The listing builds one solid part. Answer for the finished solid, in the listing's coordinates (mm). Face numbers are marked on the shaded views. A direction names the side the tool comes from. Coordinates: 2 decimals unless noted, no trailing zeros. Write each loop counter-clockwise with the first axis right and the second up, starting at its lowest first coordinate (ties: lowest second). Pieces come first, ordered by that corner, then holes.
(1) Which of the six approach directions +Z, -Z, +X, -X, +Y, -Y give full straight-line access (tool end or side, diameter ignored) to the marked faces 4, 5, 6 and 7?
(2) Given P1, Ø0.9, axis at x = 16, z = 108, coming from the -Y side; P2, Ø14.5, axis at x = -8.62, y = -7.1, coming from the +Z side; P3, Ø2, axis at x = -10.5, y = 6, coming from the +Z side, each flat-ended and moving along its own axis, determine where each tip first touches the part or whether it passes through.
(3) The part is cut by section C-C on z = 126. Determine the outline of the cut face in (x, y).
(4) Straight lines are drawn through the part: line 1 (Z direction, x = 7.5, y = -4); line 2 (X direction, y = -20.5, z = 135.5); line 3 (X direction, y = -4, z = 112). For each, find the intervals that lie inside material, in ascending order.
(5) The part is cut by section D-D on y = -18.5. Determine the outline of the cut face in (x, z).
(6) For a pull along Y with two mould halves and no side action, classify the marked faces 1, 2 and 3 as +Y half, -Y half, draft (parallel to the pull), parting line (faces both ways), or undercut.
(7) The part is cut by section B-B on x = -27.5. Determine the outline of the cut face in (y, z) (3 decimals), plus the area to 3 significant figures.
(8) The part is cut by section A-A on x = 13.5. Determine the outline of the cut face in (y, z).
from build123d import *

# Parameters (mm, degrees)
SALIENTE_EXTRUIR1_START = 2.5
SALIENTE_EXTRUIR1_DEPTH = 5
CROQUIS2_R              = 13.5
CORTAR_EXTRUIR1_DEPTH   = 3.5
CROQUIS4_R              = 4.025
SALIENTE_EXTRUIR3_DEPTH = 9
CROQUIS5_W              = 5
CROQUIS5_H              = 36
SALIENTE_EXTRUIR4_DEPTH = 38.35
CORTAR_EXTRUIR2_DEPTH   = 2
CROQUIS8_R              = 4.55
CORTAR_EXTRUIR3_DEPTH   = 67.15821583
SALIENTE_EXTRUIR5_DEPTH = 5
CORTAR_EXTRUIR4_DEPTH   = 5
SALIENTE_EXTRUIR6_START = 3.65
CROQUIS12_R             = 1
SALIENTE_EXTRUIR6_DEPTH = 3.65
SALIENTE_EXTRUIR7_START = -8.65
SALIENTE_EXTRUIR7_DEPTH = 8.65
CROQUIS14_R             = 1
CORTAR_EXTRUIR5_DEPTH   = 3.65
CROQUIS15_W             = 7.15
CROQUIS15_H             = 2.35
CORTAR_EXTRUIR6_DEPTH   = 2
CROQUIS16_W             = 7.15
CROQUIS16_H             = 2.35
SALIENTE_EXTRUIR8_DEPTH = 2
SALIENTE_EXTRUIR9_START = 2.15
CROQUIS17_R             = 1
SALIENTE_EXTRUIR9_DEPTH = 2.15
CROQUIS18_W             = 55
CROQUIS18_H             = 3
CORTAR_EXTRUIR7_DEPTH   = 3


with BuildPart() as part:
    # Croquis1 → Saliente-Extruir1 (new body)
    with BuildSketch(Plane.ZY.offset(28.973126084).offset(SALIENTE_EXTRUIR1_START)):
        with BuildLine():
            Line((108.890000566, 10.898170258), (108.890000566, -25.101829742))
            Line((108.890000566, -25.101829742), (143.890000566, -22.601829742))
            ThreePointArc((143.890000566, -22.601829742), (159.390000566, -7.101829742), (143.890000566, 8.398170258))
            Line((143.890000566, 8.398170258), (108.890000566, 10.898170258))
        make_face()
    extrude(amount=-SALIENTE_EXTRUIR1_DEPTH)

    # Croquis2 → Cortar-Extruir1 (cut)
    with BuildSketch(Plane(origin=(-26.473126084, 0, 0), x_dir=(0, 0, -1), z_dir=(1, 0, 0))):
        with Locations((-143.890000566, -7.101829742)):
            Circle(CROQUIS2_R)
    extrude(amount=-CORTAR_EXTRUIR1_DEPTH, mode=Mode.SUBTRACT)

    # Croquis4 → Saliente-Extruir3 (add)
    with BuildSketch(Plane(origin=(-29.973126084, 0, 0), x_dir=(0, 0, -1), z_dir=(1, 0, 0))):
        with Locations(Location((-143.890000566, -7.101829742, 0), (0, 0, 180))):
            Circle(CROQUIS4_R)
    extrude(amount=SALIENTE_EXTRUIR3_DEPTH)

    # Croquis5 → Saliente-Extruir4 (add)
    with BuildSketch(Plane.ZY.offset(31.473126084)):
        with Locations((106.390000566, -7.101829742)):
            Rectangle(CROQUIS5_W, CROQUIS5_H)
    extrude(amount=-SALIENTE_EXTRUIR4_DEPTH)

    # Croquis6 → Cortar-Extruir2 (cut)
    with BuildSketch(Plane.XY.offset(108.890000566)):
        with BuildLine():
            Line((-21.743906953, -10.757089493), (-16.168906615, -6.706372141))
            Line((-16.168906615, -6.706372141), (-21.289951258, -2.095098824))
            ThreePointArc((-21.289951258, -2.095098824), (-22.060016072, 1.624188646), (-18.349064321, 2.433469933))
            Line((-18.349064321, 2.433469933), (-12.053540021, -0.36926331))
            Line((-12.053540021, -0.36926331), (-10.620582506, 6.371328103))
            ThreePointArc((-10.620582506, 6.371328103), (-7.784617481, 8.89786753), (-5.228283452, 6.088729685))
            Line((-5.228283452, 6.088729685), (-4.50775949, -0.764720911))
            Line((-4.50775949, -0.764720911), (2.046242668, 1.364597186))
            ThreePointArc((2.046242668, 1.364597186), (5.652272507, 0.171849142), (4.497654785, -3.44656999))
            Line((4.497654785, -3.44656999), (-1.077345553, -7.497287342))
            Line((-1.077345553, -7.497287342), (4.04369909, -12.108560659))
            ThreePointArc((4.04369909, -12.108560659), (4.813763904, -15.827848129), (1.102812153, -16.637129416))
            Line((1.102812153, -16.637129416), (-5.192712147, -13.834396173))
            Line((-5.192712147, -13.834396173), (-6.625669661, -20.574987586))
            ThreePointArc((-6.625669661, -20.574987586), (-9.461634687, -23.101527013), (-12.017968716, -20.292389168))
            Line((-12.017968716, -20.292389168), (-12.738492677, -13.438938572))
            Line((-12.738492677, -13.438938572), (-19.292494835, -15.568256669))
            ThreePointArc((-19.292494835, -15.568256669), (-22.898524675, -14.375508625), (-21.743906953, -10.757089493))
        make_face()
    extrude(amount=-CORTAR_EXTRUIR2_DEPTH, mode=Mode.SUBTRACT)

    # Croquis8 → Cortar-Extruir3 (cut, through all)
    with BuildSketch(Plane.XY.offset(106.890000566)):
        with Locations((-8.623126084, -7.101829742)):
            Circle(CROQUIS8_R)
    extrude(amount=-CORTAR_EXTRUIR3_DEPTH, mode=Mode.SUBTRACT)

    # Croquis9 → Saliente-Extruir5 (add)
    with BuildSketch(Plane(origin=(6.876873916, 0, 0), x_dir=(0, 0, -1), z_dir=(1, 0, 0))):
        with BuildLine():
            Line((-143.890000566, -22.601829742), (-108.890000566, -25.101829742))
            Line((-108.890000566, -25.101829742), (-103.890000566, -25.101829742))
            Line((-103.890000566, -25.101829742), (-103.890000566, 10.898170258))
            Line((-103.890000566, 10.898170258), (-108.890000566, 10.898170258))
            Line((-108.890000566, 10.898170258), (-143.890000566, 8.398170258))
            ThreePointArc((-143.890000566, 8.398170258), (-159.390000566, -7.101829742), (-143.890000566, -22.601829742))
        make_face()
    extrude(amount=SALIENTE_EXTRUIR5_DEPTH)

    # Croquis11 → Cortar-Extruir4 (cut)
    with BuildSketch(Plane(origin=(11.876873916, 0, 0), x_dir=(0, 0, -1), z_dir=(1, 0, 0))):
        with BuildLine():
            Line((-153.240000566, 1.898170258), (-153.240000566, -16.101829742))
            ThreePointArc((-153.240000566, -16.101829742), (-152.844594721, -17.056423896), (-151.890000566, -17.451829742))
            Line((-151.890000566, -17.451829742), (-113.890000566, -17.451829742))
            ThreePointArc((-113.890000566, -17.451829742), (-112.935406411, -17.056423896), (-112.540000566, -16.101829742))
            Line((-112.540000566, -16.101829742), (-112.540000566, 1.898170258))
            ThreePointArc((-112.540000566, 1.898170258), (-112.935406411, 2.852764413), (-113.890000566, 3.248170258))
            Line((-113.890000566, 3.248170258), (-151.890000566, 3.248170258))
            ThreePointArc((-151.890000566, 3.248170258), (-152.844594721, 2.852764413), (-153.240000566, 1.898170258))
        make_face()
    extrude(amount=-CORTAR_EXTRUIR4_DEPTH, mode=Mode.SUBTRACT)

    # Croquis12 → Saliente-Extruir6 (add)
    with BuildSketch(Plane(origin=(11.876873916, 0, 0), x_dir=(0, 0, -1), z_dir=(1, 0, 0)).offset(SALIENTE_EXTRUIR6_START)):
        with BuildLine():
            Line((-105.390000566, -1.251829742), (-105.390000566, -3.951829742))
            Line((-105.390000566, -3.951829742), (-105.390000566, -10.251829742))
            Line((-105.390000566, -10.251829742), (-105.390000566, -12.951829742))
            Line((-105.390000566, -12.951829742), (-105.390000566, -13.601829742))
            ThreePointArc((-105.390000566, -13.601829742), (-106.268680223, -15.723150085), (-108.390000566, -16.601829742))
            Line((-108.390000566, -16.601829742), (-112.636006946, -16.601829742))
            ThreePointArc((-112.636006946, -16.601829742), (-112.564219402, -16.356396641), (-112.540000566, -16.101829742))
            Line((-112.540000566, -16.101829742), (-112.540000566, 1.898170258))
            ThreePointArc((-112.540000566, 1.898170258), (-112.564219402, 2.152737158), (-112.636006946, 2.398170258))
            Line((-112.636006946, 2.398170258), (-108.390000566, 2.398170258))
            ThreePointArc((-108.390000566, 2.398170258), (-106.268680223, 1.519490602), (-105.390000566, -0.601829742))
            Line((-105.390000566, -0.601829742), (-105.390000566, -1.251829742))
        make_face()
        with Locations((-107.494163107, -2.601829742)):
            Circle(CROQUIS12_R, mode=Mode.SUBTRACT)
        with Locations((-107.494163107, -11.601829742)):
            Circle(CROQUIS12_R, mode=Mode.SUBTRACT)
    extrude(amount=-SALIENTE_EXTRUIR6_DEPTH)

    # Croquis13 → Saliente-Extruir7 (add)
    with BuildSketch(Plane.ZY.offset(-6.876873916).offset(SALIENTE_EXTRUIR7_START)):
        with BuildLine():
            Line((153.240000566, -16.101829742), (153.240000566, 1.898170258))
            ThreePointArc((153.240000566, 1.898170258), (153.21578173, 2.152737158), (153.143994186, 2.398170258))
            Line((153.143994186, 2.398170258), (157.390000566, 2.398170258))
            ThreePointArc((157.390000566, 2.398170258), (159.51132091, 1.519490602), (160.390000566, -0.601829742))
            Line((160.390000566, -0.601829742), (160.390000566, -1.251829742))
            Line((160.390000566, -1.251829742), (160.390000566, -3.951829742))
            Line((160.390000566, -3.951829742), (160.390000566, -10.251829742))
            Line((160.390000566, -10.251829742), (160.390000566, -12.951829742))
            Line((160.390000566, -12.951829742), (160.390000566, -13.601829742))
            ThreePointArc((160.390000566, -13.601829742), (159.51132091, -15.723150085), (157.390000566, -16.601829742))
            Line((157.390000566, -16.601829742), (153.143994186, -16.601829742))
            ThreePointArc((153.143994186, -16.601829742), (153.21578173, -16.356396641), (153.240000566, -16.101829742))
        make_face()
    extrude(amount=SALIENTE_EXTRUIR7_DEPTH)

    # Croquis14 → Cortar-Extruir5 (cut)
    with BuildSketch(Plane(origin=(15.526873916, 0, 0), x_dir=(0, 0, -1), z_dir=(1, 0, 0))):
        with Locations((-158.285838025, -2.601829742)):
            Circle(CROQUIS14_R)
        with Locations((-158.285838025, -11.601829742)):
            Circle(CROQUIS14_R)
    extrude(amount=-CORTAR_EXTRUIR5_DEPTH, mode=Mode.SUBTRACT)

    # Croquis15 → Cortar-Extruir6 (cut)
    with BuildSketch(Plane(origin=(15.526873916, 0, 0), x_dir=(0, 0, -1), z_dir=(1, 0, 0))):
        with Locations((-108.965000566, -7.101829742)):
            Rectangle(CROQUIS15_W, CROQUIS15_H)
        with Locations((-156.815000566, -7.101829742)):
            Rectangle(CROQUIS15_W, CROQUIS15_H)
    extrude(amount=-CORTAR_EXTRUIR6_DEPTH, mode=Mode.SUBTRACT)

    # Croquis16 → Saliente-Extruir8 (add)
    with BuildSketch(Plane(origin=(13.526873916, 0, 0), x_dir=(0, 0, -1), z_dir=(1, 0, 0))):
        with Locations((-156.815000566, -7.101829742)):
            Rectangle(CROQUIS16_W, CROQUIS16_H)
        with Locations((-108.965000566, -7.101829742)):
            Rectangle(CROQUIS16_W, CROQUIS16_H)
    extrude(amount=SALIENTE_EXTRUIR8_DEPTH)

    # Croquis17 → Saliente-Extruir9 (add)
    # profile 1 of 2: a face of its own
    with BuildSketch(Plane(origin=(15.526873916, 0, 0), x_dir=(0, 0, -1), z_dir=(1, 0, 0)).offset(SALIENTE_EXTRUIR9_START)):
        with BuildLine():
            Line((-105.390000566, -13.601829742), (-105.390000566, -0.601829742))
            ThreePointArc((-105.390000566, -0.601829742), (-106.268680223, 1.519490602), (-108.390000566, 2.398170258))
            Line((-108.390000566, 2.398170258), (-112.636006946, 2.398170258))
            ThreePointArc((-112.636006946, 2.398170258), (-112.564219402, 2.152737158), (-112.540000566, 1.898170258))
            Line((-112.540000566, 1.898170258), (-112.540000566, -16.101829742))
            ThreePointArc((-112.540000566, -16.101829742), (-112.564219402, -16.356396641), (-112.636006946, -16.601829742))
            Line((-112.636006946, -16.601829742), (-108.390000566, -16.601829742))
            ThreePointArc((-108.390000566, -16.601829742), (-106.268680223, -15.723150085), (-105.390000566, -13.601829742))
        make_face()
        with Locations((-107.494163107, -11.601829742)):
            Circle(CROQUIS17_R, mode=Mode.SUBTRACT)
        with Locations((-107.494163107, -2.601829742)):
            Circle(CROQUIS17_R, mode=Mode.SUBTRACT)
    # profile 2 of 2: a face of its own
    with BuildSketch(Plane(origin=(15.526873916, 0, 0), x_dir=(0, 0, -1), z_dir=(1, 0, 0)).offset(SALIENTE_EXTRUIR9_START)):
        with BuildLine():
            Line((-160.390000566, -0.601829742), (-160.390000566, -13.601829742))
            ThreePointArc((-160.390000566, -13.601829742), (-159.51132091, -15.723150085), (-157.390000566, -16.601829742))
            Line((-157.390000566, -16.601829742), (-153.143994186, -16.601829742))
            ThreePointArc((-153.143994186, -16.601829742), (-153.21578173, -16.356396641), (-153.240000566, -16.101829742))
            Line((-153.240000566, -16.101829742), (-153.240000566, 1.898170258))
            ThreePointArc((-153.240000566, 1.898170258), (-153.21578173, 2.152737158), (-153.143994186, 2.398170258))
            Line((-153.143994186, 2.398170258), (-157.390000566, 2.398170258))
            ThreePointArc((-157.390000566, 2.398170258), (-159.51132091, 1.519490602), (-160.390000566, -0.601829742))
        make_face()
        with Locations((-158.285838025, -11.601829742)):
            Circle(CROQUIS17_R, mode=Mode.SUBTRACT)
        with Locations((-158.285838025, -2.601829742)):
            Circle(CROQUIS17_R, mode=Mode.SUBTRACT)
    extrude(amount=-SALIENTE_EXTRUIR9_DEPTH)

    # Croquis18 → Cortar-Extruir7 (cut)
    with BuildSketch(Plane(origin=(17.676873916, 0, 0), x_dir=(0, 0, -1), z_dir=(1, 0, 0))):
        with Locations((-132.890000566, -7.101829742)):
            Rectangle(CROQUIS18_W, CROQUIS18_H)
    extrude(amount=-CORTAR_EXTRUIR7_DEPTH, mode=Mode.SUBTRACT)


solid = part.part
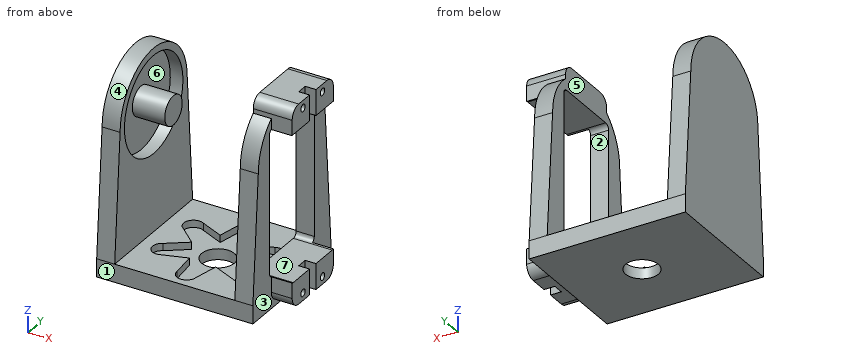
Model answer:
1. face 4: +Z, -X
1. face 5: +Z, +Y, -Y
1. face 6: none
1. face 7: +X
2. P1: stops at y = -16.6
2. P2: stops at z = 106.89
2. P3: stops at z = 108.89
3. outline: (-31.47, -23.88) - (-26.47, -23.88) - (-26.47, 9.68) - (-31.47, 9.68) - close; (6.88, -23.88) - (11.88, -23.88) - (11.88, -17.45) - (6.88, -17.45) - close; (6.88, 3.25) - (11.88, 3.25) - (11.88, 9.68) - (6.88, 9.68) - close
4. line 1: z = 103.89 to 112.54, 153.24 to 160.39
4. line 2: x = -31.47 to -26.47, 6.88 to 11.88
4. line 3: x = -31.47 to -26.47, 6.88 to 17.68
5. outline: (-31.47, 103.89) - (11.88, 103.89) - (11.88, 154.39) - (6.88, 154.39) - (6.88, 108.89) - (-6.18, 108.89) - (-6.18, 106.89) - (-12.21, 106.89) - (-12.21, 108.89) - (-26.47, 108.89) - (-26.47, 136.66) - (-29.97, 136.66) - (-29.97, 151.12) - (-26.47, 151.12) - (-26.47, 154.39) - (-31.47, 154.39) - close
6. face 1: -Y half
6. face 2: undercut
6. face 3: draft
7. outline: (-25.102, 103.89) - (10.898, 103.89) - (10.898, 108.89) - (8.398, 143.89) arc R15.5 ccw to (-22.602, 143.89) - (-25.102, 108.89) - close; circle Ø8.05 at (-7.102, 143.89); hole circle Ø27 at (-7.102, 143.89)
7. area: 1,210 mm2
8. outline: (-16.6, 108.39) arc R3 ccw to (-13.6, 105.39) - (-0.6, 105.39) arc R3 ccw to (2.4, 108.39) - (2.4, 112.64) arc R1.35 cw to (1.9, 112.54) - (-16.1, 112.54) arc R1.35 cw to (-16.6, 112.64) - close; (-16.6, 153.14) arc R1.35 cw to (-16.1, 153.24) - (1.9, 153.24) arc R1.35 cw to (2.4, 153.14) - (2.4, 157.39) arc R3 ccw to (-0.6, 160.39) - (-13.6, 160.39) arc R3 ccw to (-16.6, 157.39) - close; hole circle Ø2 at (-11.6, 107.49); hole circle Ø2 at (-11.6, 158.29); hole circle Ø2 at (-2.6, 107.49); hole circle Ø2 at (-2.6, 158.29)
